```python
from build123d import *
from OCP.BRepFilletAPI import BRepFilletAPI_MakeChamfer

# Parameters (mm, degrees)
SKETCH1_W           = 88.5
SKETCH1_H           = 88.5
BOSS_EXTRUDE1_DEPTH = 4
SKETCH1_3_W         = 88.5
SKETCH1_3_H         = 88.5
SKETCH1_3_W_2       = 80.5
SKETCH1_3_H_2       = 80.5
SKETCH1_3_R         = 3.5
SKETCH1_3_R_2       = 1.5
BOSS_EXTRUDE2_DEPTH = 9
CHAMFER1_SIZE       = 0.5
CHAMFER1_SIZE2      = 1.866025404
SKETCH4_W           = 88.5
SKETCH4_H           = 88.5
SKETCH4_W_2         = 80.5
SKETCH4_H_2         = 80.5
BOSS_EXTRUDE3_DEPTH = 39
SKETCH5_R           = 6.5
CUT_EXTRUDE1_DEPTH  = 16
FILLET1_R           = 2
FILLET2_R           = 2
FILLET3_R           = 2
FILLET4_R           = 2
FILLET5_R           = 2
FILLET6_R           = 2
FILLET7_R           = 2
CUT_EXTRUDE2_DEPTH  = 10
SKETCH9_W           = 28
SKETCH9_H           = 38.5
CUT_EXTRUDE3_DEPTH  = 88.5
SKETCH13_R          = 1.6
CUT_EXTRUDE5_DEPTH  = 10
SKETCH14_W          = 2
SKETCH14_H          = 3
CUT_EXTRUDE6_DEPTH  = 48
SKETCH15_W          = 2
SKETCH15_H          = 3
CUT_EXTRUDE7_DEPTH  = 48
SKETCH16_W          = 80.5
SKETCH16_H          = 3
CUT_EXTRUDE8_DEPTH  = 2


with BuildPart() as part:
    # Sketch1 → Boss-Extrude1 (new body)
    with BuildSketch(Plane(origin=(0, 0, 0), x_dir=(0, 1, 0), z_dir=(0, 0, 1))):
        Rectangle(SKETCH1_W, SKETCH1_H)
    extrude(amount=-BOSS_EXTRUDE1_DEPTH)

    # Sketch1_3 → Boss-Extrude2 (add)
    # profile 1 of 4: a face of its own
    with BuildSketch(Plane(origin=(0, 0, 0), x_dir=(0, 1, 0), z_dir=(0, 0, 1))):
        Rectangle(SKETCH1_3_W, SKETCH1_3_H)
        Rectangle(SKETCH1_3_W_2, SKETCH1_3_H_2, mode=Mode.SUBTRACT)
    # profile 2 of 4: a face of its own
    with BuildSketch(Plane(origin=(0, 0, 0), x_dir=(0, 1, 0), z_dir=(0, 0, 1))):
        with Locations(Location((7.75, -26, 0), (0, 0, 90))):
            Circle(SKETCH1_3_R)
        with Locations(Location((7.75, -26, 0), (0, 0, 270))):
            Circle(SKETCH1_3_R_2, mode=Mode.SUBTRACT)
    # profile 3 of 4: a face of its own
    with BuildSketch(Plane(origin=(0, 0, 0), x_dir=(0, 1, 0), z_dir=(0, 0, 1))):
        with Locations(Location((34.25, 14.25, 0), (0, 0, 90))):
            Circle(SKETCH1_3_R)
        with Locations(Location((34.25, 14.25, 0), (0, 0, 270))):
            Circle(SKETCH1_3_R_2, mode=Mode.SUBTRACT)
    # profile 4 of 4: a face of its own
    with BuildSketch(Plane(origin=(0, 0, 0), x_dir=(0, 1, 0), z_dir=(0, 0, 1))):
        with Locations(Location((-34.25, 14.25, 0), (0, 0, 90))):
            Circle(SKETCH1_3_R)
        with Locations(Location((-34.25, 14.25, 0), (0, 0, 270))):
            Circle(SKETCH1_3_R_2, mode=Mode.SUBTRACT)
    extrude(amount=BOSS_EXTRUDE2_DEPTH)

    # Chamfer1: one chamfer whose edges measure the first distance from different faces: ONE call of the kernel's chamfer builder (chamfer() names one face for all edges)
    chamfer1_edges_1 = [part.edges().sort_by_distance(p)[0] for p in [
        (24.5, 7.75, 9),
    ]]
    chamfer1_side_1 = [part.faces().sort_by_distance(p)[0] for p in [
        (29.401005051, 7.75, 9),
    ]]
    chamfer1_edges_2 = [part.edges().sort_by_distance(p)[0] for p in [
        (-15.75, 34.25, 9),
    ]]
    chamfer1_side_2 = [part.faces().sort_by_distance(p)[0] for p in [
        (-10.848994949, 34.25, 9),
    ]]
    chamfer1_edges_3 = [part.edges().sort_by_distance(p)[0] for p in [
        (-15.75, -34.25, 9),
    ]]
    chamfer1_side_3 = [part.faces().sort_by_distance(p)[0] for p in [
        (-10.848994949, -34.25, 9),
    ]]
    chamfer1 = BRepFilletAPI_MakeChamfer(part.part.solid().wrapped)
    for e in chamfer1_edges_1:
        chamfer1.Add(CHAMFER1_SIZE, CHAMFER1_SIZE2, e.wrapped, chamfer1_side_1[0].wrapped)  # the first distance lies on this face
    for e in chamfer1_edges_2:
        chamfer1.Add(CHAMFER1_SIZE, CHAMFER1_SIZE2, e.wrapped, chamfer1_side_2[0].wrapped)  # the first distance lies on this face
    for e in chamfer1_edges_3:
        chamfer1.Add(CHAMFER1_SIZE, CHAMFER1_SIZE2, e.wrapped, chamfer1_side_3[0].wrapped)  # the first distance lies on this face
    add(Compound.cast(chamfer1.Shape()), mode=Mode.REPLACE)

    # Sketch4 → Boss-Extrude3 (add)
    with BuildSketch(Plane.XY.offset(9)):
        Rectangle(SKETCH4_W, SKETCH4_H)
        Rectangle(SKETCH4_W_2, SKETCH4_H_2, mode=Mode.SUBTRACT)
    extrude(amount=BOSS_EXTRUDE3_DEPTH)

    # Sketch5 → Cut-Extrude1 (cut)
    with BuildSketch(Plane.XZ.offset(44.25)):
        with Locations((-26.25, 24)):
            Circle(SKETCH5_R)
        with BuildLine():
            Line((7.25, 30), (13.25, 30))
            ThreePointArc((13.25, 30), (14.664213562, 29.414213562), (15.25, 28))
            Line((15.25, 28), (15.25, 26))
            ThreePointArc((15.25, 26), (14.664213562, 24.585786438), (13.25, 24))
            Line((13.25, 24), (7.25, 24))
            ThreePointArc((7.25, 24), (5.835786438, 24.585786438), (5.25, 26))
            Line((5.25, 26), (5.25, 28))
            ThreePointArc((5.25, 28), (5.835786438, 29.414213562), (7.25, 30))
        make_face()
        with BuildLine():
            Line((-10.75, 17), (-4.67, 17))
            ThreePointArc((-4.67, 17), (-3.255786438, 16.414213562), (-2.67, 15))
            Line((-2.67, 15), (-2.67, 13))
            ThreePointArc((-2.67, 13), (-3.255786438, 11.585786438), (-4.67, 11))
            Line((-4.67, 11), (-10.75, 11))
            ThreePointArc((-10.75, 11), (-12.164213562, 11.585786438), (-12.75, 13))
            Line((-12.75, 13), (-12.75, 15))
            ThreePointArc((-12.75, 15), (-12.164213562, 16.414213562), (-10.75, 17))
        make_face()
    extrude(amount=-CUT_EXTRUDE1_DEPTH, mode=Mode.SUBTRACT)

    # Fillet1
    fillet1_edges = [part.edges().sort_by_distance(p)[0] for p in [
        (44.25, -44.25, 22),
    ]]
    fillet(fillet1_edges, radius=FILLET1_R)

    # Fillet2
    fillet2_edges = [part.edges().sort_by_distance(p)[0] for p in [
        (-44.25, -44.25, 22),
    ]]
    fillet(fillet2_edges, radius=FILLET2_R)

    # Fillet3
    fillet3_edges = [part.edges().sort_by_distance(p)[0] for p in [
        (44.25, 44.25, 22),
    ]]
    fillet(fillet3_edges, radius=FILLET3_R)

    # Fillet4
    fillet4_edges = [part.edges().sort_by_distance(p)[0] for p in [
        (-44.25, 44.25, 22),
    ]]
    fillet(fillet4_edges, radius=FILLET4_R)

    # Fillet5
    fillet5_edges = [part.edges().sort_by_distance(p)[0] for p in [
        (29.5, 7.75, 0),
    ]]
    fillet(fillet5_edges, radius=FILLET5_R)

    # Fillet6
    fillet6_edges = [part.edges().sort_by_distance(p)[0] for p in [
        (-10.75, -34.25, 0),
    ]]
    fillet(fillet6_edges, radius=FILLET6_R)

    # Fillet7
    fillet7_edges = [part.edges().sort_by_distance(p)[0] for p in [
        (-10.75, 34.25, 0),
    ]]
    fillet(fillet7_edges, radius=FILLET7_R)

    # Sketch6 → Cut-Extrude2 (cut)
    with BuildSketch(Plane(origin=(-44.25, 0, 0), x_dir=(0, -1, 0), z_dir=(-1, 0, 0))):
        with BuildLine():
            Line((36, 1.25), (35, 1.25))
            ThreePointArc((35, 1.25), (34.292893219, 1.542893219), (34, 2.25))
            Line((34, 2.25), (34, 41.75))
            ThreePointArc((34, 41.75), (34.292893219, 42.457106781), (35, 42.75))
            Line((35, 42.75), (36, 42.75))
            ThreePointArc((36, 42.75), (36.707106781, 42.457106781), (37, 41.75))
            Line((37, 41.75), (37, 2.25))
            ThreePointArc((37, 2.25), (36.707106781, 1.542893219), (36, 1.25))
        make_face()
        with BuildLine():
            Line((31, 2.25), (31, 41.75))
            ThreePointArc((31, 41.75), (30.707106781, 42.457106781), (30, 42.75))
            Line((30, 42.75), (29, 42.75))
            ThreePointArc((29, 42.75), (28.292893219, 42.457106781), (28, 41.75))
            Line((28, 41.75), (28, 2.25))
            ThreePointArc((28, 2.25), (28.292893219, 1.542893219), (29, 1.25))
            Line((29, 1.25), (30, 1.25))
            ThreePointArc((30, 1.25), (30.707106781, 1.542893219), (31, 2.25))
        make_face()
        with BuildLine():
            Line((25, 2.25), (25, 41.75))
            ThreePointArc((25, 41.75), (24.707106781, 42.457106781), (24, 42.75))
            Line((24, 42.75), (23, 42.75))
            ThreePointArc((23, 42.75), (22.292893219, 42.457106781), (22, 41.75))
            Line((22, 41.75), (22, 2.25))
            ThreePointArc((22, 2.25), (22.292893219, 1.542893219), (23, 1.25))
            Line((23, 1.25), (24, 1.25))
            ThreePointArc((24, 1.25), (24.707106781, 1.542893219), (25, 2.25))
        make_face()
        with BuildLine():
            Line((19, 2.25), (19, 41.75))
            ThreePointArc((19, 41.75), (18.707106781, 42.457106781), (18, 42.75))
            Line((18, 42.75), (17, 42.75))
            ThreePointArc((17, 42.75), (16.292893219, 42.457106781), (16, 41.75))
            Line((16, 41.75), (16, 2.25))
            ThreePointArc((16, 2.25), (16.292893219, 1.542893219), (17, 1.25))
            Line((17, 1.25), (18, 1.25))
            ThreePointArc((18, 1.25), (18.707106781, 1.542893219), (19, 2.25))
        make_face()
        with BuildLine():
            Line((13, 2.25), (13, 41.75))
            ThreePointArc((13, 41.75), (12.707106781, 42.457106781), (12, 42.75))
            Line((12, 42.75), (11, 42.75))
            ThreePointArc((11, 42.75), (10.292893219, 42.457106781), (10, 41.75))
            Line((10, 41.75), (10, 2.25))
            ThreePointArc((10, 2.25), (10.292893219, 1.542893219), (11, 1.25))
            Line((11, 1.25), (12, 1.25))
            ThreePointArc((12, 1.25), (12.707106781, 1.542893219), (13, 2.25))
        make_face()
        with BuildLine():
            Line((7, 2.25), (7, 41.75))
            ThreePointArc((7, 41.75), (6.707106781, 42.457106781), (6, 42.75))
            Line((6, 42.75), (5, 42.75))
            ThreePointArc((5, 42.75), (4.292893219, 42.457106781), (4, 41.75))
            Line((4, 41.75), (4, 2.25))
            ThreePointArc((4, 2.25), (4.292893219, 1.542893219), (5, 1.25))
            Line((5, 1.25), (6, 1.25))
            ThreePointArc((6, 1.25), (6.707106781, 1.542893219), (7, 2.25))
        make_face()
    extrude(amount=-CUT_EXTRUDE2_DEPTH, mode=Mode.SUBTRACT)

    # Sketch9 → Cut-Extrude3 (cut)
    with BuildSketch(Plane.ZY.offset(44.25)):
        with Locations((34, 25)):
            Rectangle(SKETCH9_W, SKETCH9_H)
    extrude(amount=-CUT_EXTRUDE3_DEPTH, mode=Mode.SUBTRACT)

    # Sketch13 → Cut-Extrude5 (cut)
    with BuildSketch(Plane(origin=(0, 0, -4), x_dir=(1, 0, 0), z_dir=(0, 0, -1))):
        with Locations(Location((-25.61, 28, 0), (0, 0, 180))):
            Circle(SKETCH13_R)
        with Locations(Location((10.19, 28, 0), (0, 0, 180))):
            Circle(SKETCH13_R)
        with Locations(Location((-25.61, -28, 0), (0, 0, 180))):
            Circle(SKETCH13_R)
        with Locations(Location((10.19, -28, 0), (0, 0, 180))):
            Circle(SKETCH13_R)
    extrude(amount=-CUT_EXTRUDE5_DEPTH, mode=Mode.SUBTRACT)

    # Sketch14 → Cut-Extrude6 (cut)
    with BuildSketch(Plane(origin=(0, 5.75, 0), x_dir=(-1, 0, 0), z_dir=(0, 1, 0))):
        with Locations((-41.25, 44.5)):
            Rectangle(SKETCH14_W, SKETCH14_H)
    extrude(amount=-CUT_EXTRUDE6_DEPTH, mode=Mode.SUBTRACT)

    # Sketch15 → Cut-Extrude7 (cut)
    with BuildSketch(Plane(origin=(0, 5.75, 0), x_dir=(-1, 0, 0), z_dir=(0, 1, 0))):
        with Locations((41.25, 44.5)):
            Rectangle(SKETCH15_W, SKETCH15_H)
    extrude(amount=-CUT_EXTRUDE7_DEPTH, mode=Mode.SUBTRACT)

    # Sketch16 → Cut-Extrude8 (cut)
    with BuildSketch(Plane(origin=(0, -40.25, 0), x_dir=(-1, 0, 0), z_dir=(0, 1, 0))):
        with Locations((0, 44.5)):
            Rectangle(SKETCH16_W, SKETCH16_H)
    extrude(amount=-CUT_EXTRUDE8_DEPTH, mode=Mode.SUBTRACT)


solid = part.part
```
Design review of the part built by this model. Coordinates are the model's own, in mm. A direction names the side the tool comes from. Give positions to 0.01 mm unless a question says otherwise; leave off trailing zeros. Loops run counter-clockwise (first coordinate to the right, second up) from the corner with the lowest first, then second, coordinate; pieces in that order, holes last. Notation, with made-up numbers: (-17, 4) -> (5, 4) arc R11 cw to (5, 25) -> close; hole circle Ø10 at (-6.5, 55). An arc over 180 degrees is marked (long way). Write each question's results on one line, items separated by ' | '.
Q1. The part is to be moulded in two halves that separate along Y. For faces 6 (the face through (-1, -1, 0)), 7 (the face through (1, -42.25, 45)), 8 (the face through (44.25, -10, 16)), 9 (the face through (-42, -19, 22)), say which applies: +Y half, -Y half, draft (parallel to the pull), parting line (faces both ways), or undercut.
Reply:
face 6: undercut | face 7: +Y half | face 8: draft | face 9: undercut
Q2. Machinability: for faces 1 (the face through (10, -42, 30)), 2 (the face through (10.398, -26.414, -2.028)), 3 (the face through (-14, 34, 0)), 4 (the face through (0, 41, 20)), 5 (the face through (-42, -31, 22)), which of the approach directions +Z, -Z, +X, -X, +Y, -Y give a long, thin tool a straight path to every point of the face, cutting with its end or side? Answer none if there is none.
Reply:
face 1: +Y, -Y | face 2: +Z, -Z | face 3: +Z | face 4: +Z, +X, -X, +Y | face 5: -X
Q3. Take a section at A-A, the plane x = 26. Write out the cut boundary in (y, z), plus the area to 3 significant figures.
Reply:
outline: (-44.25, -4) -> (44.25, -4) -> (44.25, 20) -> (40.25, 20) -> (40.25, 0) -> (13.25, 0) arc R2 cw to (11.25, 2) -> (11.25, 9) -> (9.75, 9) -> (9.25, 7.13) -> (9.25, 0) -> (6.25, 0) -> (6.25, 7.13) -> (5.75, 9) -> (4.25, 9) -> (4.25, 2) arc R2 cw to (2.25, 0) -> (-40.25, 0) -> (-40.25, 43) -> (-42.25, 43) -> (-42.25, 46) -> (-40.25, 46) -> (-40.25, 48) -> (-44.25, 48) -> close | area: 657 mm²
Q4. Wall thickness on L1, parallel to Y at x = 26, z = 1.75; L2, parallel to Y at x = -25.61, z = -1.55; L3, parallel to Y at x = 26, z = 4: over which ranges is each line inside the solid? List them lowest first.
Reply:
L1: y = -44.25 to -40.25, 4.23 to 6.25, 9.25 to 11.27, 40.25 to 44.25 | L2: y = -44.25 to -29.6, -26.4 to 26.4, 29.6 to 44.25 | L3: y = -44.25 to -40.25, 4.25 to 6.25, 9.25 to 11.25, 40.25 to 44.25
Q5. Take a section at D-D, the plane z = 22.5. Give the number of separate pieces and of enclosed holes in the cut face, plus the area to 3 significant figures.
Reply:
separate pieces: 8 | enclosed holes: 0 | area: 598 mm²
Q6. Take a section at B-B, the plane x = -25.61. Write out the cut boundary in (y, z).
Reply:
outline: (-44.25, -4) -> (-29.6, -4) -> (-29.6, 0) -> (-40.25, 0) -> (-40.25, 17.53) -> (-44.25, 17.53) -> close; (-44.25, 30.47) -> (-40.25, 30.47) -> (-40.25, 43) -> (-42.25, 43) -> (-42.25, 46) -> (-40.25, 46) -> (-40.25, 48) -> (-44.25, 48) -> close; (-26.4, -4) -> (26.4, -4) -> (26.4, 0) -> (-26.4, 0) -> close; (29.6, -4) -> (44.25, -4) -> (44.25, 20) -> (40.25, 20) -> (40.25, 0) -> (29.6, 0) -> close
Q7. Take a section at C-C, the plane y = 34.25. Write out the cut boundary in (x, z).
Reply:
outline: (-44.25, -4) -> (44.25, -4) -> (44.25, 20) -> (40.25, 20) -> (40.25, 0) -> (-8.75, 0) arc R2 cw to (-10.75, 2) -> (-10.75, 9) -> (-12.25, 9) -> (-12.75, 7.13) -> (-12.75, 0) -> (-15.75, 0) -> (-15.75, 7.13) -> (-16.25, 9) -> (-17.75, 9) -> (-17.75, 2) arc R2 cw to (-19.75, 0) -> (-40.25, 0) -> (-40.25, 20) -> (-44.25, 20) -> close
Q8. For pin 1 Ø1.5 at (x, z) = (15.5, 44) entering from +Y; pin 2 Ø4 at (x, y) = (-25.61, -28) entering from +Z; pin 3 Ø1.5 at (x, z) = (-20.5, 29) entering from +Y, all flat-tipped, find the tip position at first contact; note any pin that passes through.
Reply:
pin 1: stops at y = -42.25 | pin 2: stops at z = 0 | pin 3: stops at y = -40.25
